Input: part model. Units: mm. Frame: model coordinates. A direction names the side the tool comes from. Coordinates: 2 decimals unless noted, no trailing zeros. Order: outer loops, then holes, each group sorted by start corner. A loop starts at its lowest first (then second) coordinate and runs counter-clockwise, first axis right, second up. Notation, with made-up numbers: (-24, 54) -> (-10, 54) arc R18 cw to (-10, 67) -> close; hole circle Ø9 at (9.25, 47.5). An arc over 180 degrees is marked (long way). Answer as CSV lines item,"result".
Autodesk Inventor part; units mm, degrees
ref_plane "YZ Plane" through (0, 0, 0) normal (1, 0, 0) x (0, 1, 0)
ref_plane "XZ Plane" through (0, 0, 0) normal (0, 1, 0) x (-1, 0, 0)
ref_plane "XY Plane" through (0, 0, 0) normal (0, 0, 1) x (1, 0, 0)
sketch "Sketch1" plane through (0, 0, 0) normal (0, 0, 1) x (1, 0, 0)
  arc A0 (187.325, 0) -> (0, 187.325) centre (0, 0) ccw
  arc A1 (136.525, 0) -> (0, 136.525) centre (0, 0) ccw
  line L0 (0, 136.525) -> (0, 187.325)
  line L1 (136.525, 0) -> (187.325, 0)
  point P0 (161.925, 0)
  point P1 (0, 161.925)
  dimension "d2" = 187.325
  dimension "d3" = 136.525
extrude "Extrusion1" add sketch "Sketch1" along normal blind 0.4
sketch "Sketch3" plane through (0, 0, 0.4) normal (0, 0, 1) x (1, 0, 0)
  line L0 (179.9922, 39.0399) -> (181.231, 32.8119)
  arc A0 (178.117, 32.1925) -> (181.231, 32.8119) centre (179.674, 32.5022) ccw
  line L1 (178.117, 32.1925) -> (176.8782, 38.4205)
  arc A1 (179.9922, 39.0399) -> (176.8782, 38.4205) centre (178.4352, 38.7302) ccw
  arc A2 (130.2137, 125.7236) -> (132.4588, 127.9686) centre (131.3362, 126.8461) ccw
  line L2 (127.9686, 132.4588) -> (132.4588, 127.9686)
  arc A3 (127.9686, 132.4588) -> (125.7236, 130.2137) centre (126.8461, 131.3362) ccw
  line L3 (130.2137, 125.7236) -> (125.7236, 130.2137)
  line L4 (32.8119, 181.231) -> (39.0399, 179.9922)
  arc A4 (38.4205, 176.8782) -> (39.0399, 179.9922) centre (38.7302, 178.4352) ccw
  line L5 (38.4205, 176.8782) -> (32.1925, 178.117)
  arc A5 (32.8119, 181.231) -> (32.1925, 178.117) centre (32.5022, 179.674) ccw
  circle A6 centre (90.0738, 130.599) radius 5.334
  circle A7 centre (158.6401, 1.6445) radius 5.334
  point P0 (0, 0)
extrude "Extrusion2" cut sketch "Sketch3" against normal through all
properties part number "3DPRINT,CABLE,TRAY" material "ABS Plastic"
1. Reachability of faces 1 (the face through (130.18, 130.25, 0.2)), 2 (the face through (131, 133.9, 0.2)) from +Z, -Z, +X, -X, +Y, -Y: full face, straight path, thin tool, end or side. Return the list, or none.
Findings:
face 1,"+Z, -Z"
face 2,"+Z, -Z, +X, +Y"
2. Cut plane D-D (x = 109.5). Return the cut outline in (y, z).
Findings:
outline,"(81.54, 0) -> (151.99, 0) -> (151.99, 0.4) -> (81.54, 0.4) -> close"
3. Cut plane C-C (y = 151.5). Return the cut outline in (x, z).
Findings:
outline,"(0, 0) -> (110.17, 0) -> (110.17, 0.4) -> (0, 0.4) -> close"
4. Mould query, pull axis Y, two halves, no side actions, for faces 3 (the face through (92, 116, 0.4)), 4 (the face through (128, 127.94, 0.2)), 5 (the face through (95.47, 97.593, 0.197)). Classes: released by +Y, released by -Y, zero draft, split by the parting line, or undercut.
Findings:
face 3,"zero draft"
face 4,"undercut"
face 5,"released by -Y"
5. Contact query for a flat-ended pin moving along its axis: pin 1 (14 mm diameter, centred on x = 158.64, y = 1.64, fed in from +Z). Output: stop coordinate, or through.
Findings:
pin 1,"stops at z = 0.4"
6. Cut plane B-B (z = 0.2). State how many separate pieces and enclosed holes the cut face has, plus the area to 3 significant figures.
Findings:
separate pieces,"1"
enclosed holes,"4"
area,"12,700 mm2"
7. Cut plane A-A (x = 88). Return the cut outline in (y, z), plus the area to 3 significant figures.
Findings:
outline,"(104.38, 0) -> (125.68, 0) -> (125.68, 0.4) -> (104.38, 0.4) -> close; (135.51, 0) -> (165.37, 0) -> (165.37, 0.4) -> (135.51, 0.4) -> close"
area,"20.5 mm2"
8. Ray query, line 1 along Y through (x, z) = (31.5, 0.35); line 2 along Y through (x, z) = (94.5, 0.3); line 3 along X through (y, z) = (27, 0.15). Return the intervals inside material, ascending.
Findings:
line 1,"y = 132.84 to 178.44, 180.91 to 184.66"
line 2,"y = 98.53 to 127.62, 133.58 to 161.74"
line 3,"x = 133.83 to 185.37"
